Answer from the drawing. Dimensions are ordinates in mm from the lowest x, y and z of the part. A direction names the side the tool comes from. Round coordinates to 2 decimals unless told otherwise and drop trailing zeros. Write each loop counter-clockwise with the first axis right and the second up, starting at its lowest first coordinate (ties: lowest second). Pieces come first, ordered by that corner, then holes. Notation, with made-up numbers: (-0.5, 5.5) - (14.5, 5.5) arc R28 cw to (14.5, 23.5) - close; hole circle Ø5 at (52.25, 23.5). An arc over 180 degrees is marked (long way). Answer in a Markdown table with one row per item.
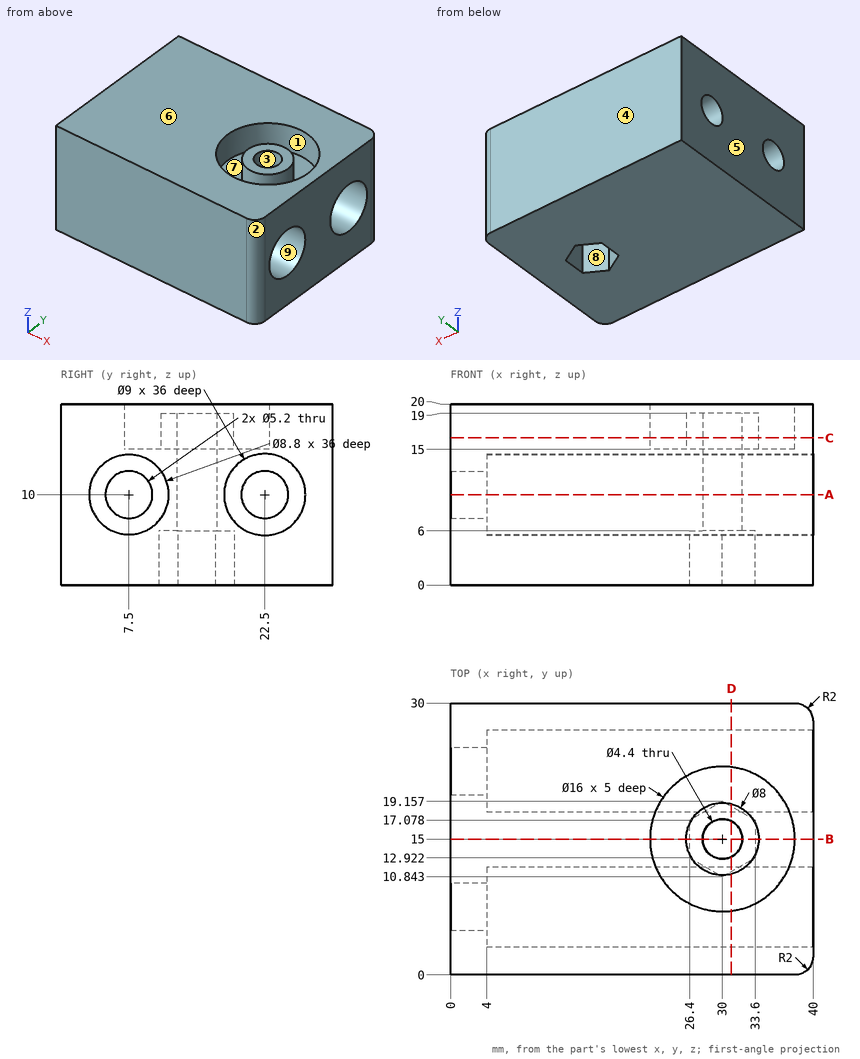
(1) Find the intervals of material crossed by line 1 (Z direction, x = 14.5, y = 7.5); line 2 (X direction, y = 11.5, z = 16.25) (1 decimal); line 3 (Y direction, x = 22.5, z = 12.5), in increasing order.
Checked values:
| item | result |
|---|---|
| line 1 | z = 0 to 5.6, 14.4 to 20 |
| line 2 | x = 0 to 22.8, 28.1 to 31.9, 37.2 to 40 |
| line 3 | y = 0 to 3.88, 11.12 to 18.76, 26.24 to 30 |
(2) Section C-C (z = 16.25) is taken. Give the vertices of the cut face in (x, y), and give its area (3 significant figures).
Checked values:
| item | result |
|---|---|
| outline | (0, 0) - (38, 0) arc R2 ccw to (40, 2) - (40, 28) arc R2 ccw to (38, 30) - (0, 30) - close; circle Ø8 at (30, 15); hole circle Ø16 at (30, 15); hole circle Ø4.4 at (30, 15) |
| area | 1,030 mm2 |
(3) Flat-ended cylindrical pins translate along their axes: pin 1 (2.5 mm diameter, centred on y = 20.5, z = 10.5, fed in from +X); pin 2 (2.5 mm diameter, centred on x = 30, y = 15, fed in from +Z); pin 3 (3.5 mm diameter, centred on x = 30.5, y = 14.5, fed in from -Z); pin 4 (8 mm diameter, centred on x = 32, y = 15.5, fed in from +Z). Find the tip coordinate at first contact, or state that the pin passes through.
Checked values:
| item | result |
|---|---|
| pin 1 | stops at x = 4 |
| pin 2 | passes through |
| pin 3 | stops at z = 6 |
| pin 4 | stops at z = 19 |
(4) For a pull along X with two mould halves and no side action, classify the marked faces 1, 2, 3 and 4 as pulls with the +X half, pulls with the -X half, needs draft (parallel to the pull), parting line crosses it, or undercut.
Checked values:
| item | result |
|---|---|
| face 1 | undercut |
| face 2 | pulls with the +X half |
| face 3 | undercut |
| face 4 | needs draft |
(5) Section B-B (y = 15) is taken. Give the vertices of the cut face in (x, z).
Checked values:
| item | result |
|---|---|
| outline | (0, 0) - (26.4, 0) - (26.4, 6) - (27.8, 6) - (27.8, 19) - (26, 19) - (26, 15) - (22, 15) - (22, 20) - (0, 20) - close; (32.2, 6) - (33.6, 6) - (33.6, 0) - (40, 0) - (40, 20) - (38, 20) - (38, 15) - (34, 15) - (34, 19) - (32.2, 19) - close |
(6) Section A-A (z = 10) is taken. Give the vertices of the cut face in (x, y).
Checked values:
| item | result |
|---|---|
| outline | (0, 0) - (38, 0) arc R2 ccw to (40, 2) - (40, 3.1) - (4, 3.1) - (4, 4.9) - (0, 4.9) - close; (0, 10.1) - (4, 10.1) - (4, 11.9) - (40, 11.9) - (40, 18) - (4, 18) - (4, 19.9) - (0, 19.9) - close; (0, 25.1) - (4, 25.1) - (4, 27) - (40, 27) - (40, 28) arc R2 ccw to (38, 30) - (0, 30) - close; hole circle Ø4.4 at (30, 15) |
(7) Section D-D (x = 31) is taken. Give the vertices of the cut face in (y, z).
Checked values:
| item | result |
|---|---|
| outline | (0, 0) - (11.42, 0) - (11.42, 6) - (13.04, 6) - (13.04, 19) - (11.13, 19) - (11.13, 15) - (7.06, 15) - (7.06, 20) - (0, 20) - close; (16.96, 6) - (18.58, 6) - (18.58, 0) - (30, 0) - (30, 20) - (22.94, 20) - (22.94, 15) - (18.87, 15) - (18.87, 19) - (16.96, 19) - close; hole circle Ø8.8 at (7.5, 10); hole circle Ø9 at (22.5, 10) |
(8) For the marked faces 5, 6, 7, 8 and 9, determine the directions among +Z, -Z, +X, -X, +Y, -Y from which every point of the face is accessible in a straight line to the end or side of a thin tool.
Checked values:
| item | result |
|---|---|
| face 5 | +Z, -Z, -X, +Y, -Y |
| face 6 | +Z, +X, -X, +Y, -Y |
| face 7 | +Z |
| face 8 | -Z |
| face 9 | +X |
